CAD build for the part. Positions are in the model's coordinates, mm. A direction names the side the tool comes from. Coordinates: 2 decimals unless noted, no trailing zeros. Order: outer loops, then holes, each group sorted by start corner. A loop starts at its lowest first (then second) coordinate and runs counter-clockwise, first axis right, second up. Notation, with made-up numbers: (40, -16.5) - (68, -16.5) arc R24 ccw to (68, 6.5) - close; hole circle Ø10 at (76.5, 43). An arc over 180 degrees is marked (long way). Return JSON: item names as keys, results as strings.
from build123d import *

# Parameters (mm, degrees)
F1_DEPTH     = 58.3
F3_DEPTH     = 9.017
F4_W         = 5.08
F4_H         = 2.54
F5_DEPTH     = 50.801
F6_T1_DEPTH  = 17.9471724254
F6_T3_DEPTH  = 16.9545
F6_T5_DEPTH  = 52.07
F6_T7_DEPTH  = 22.3848784961
F6_T9_DEPTH  = 12.2248784961
F6_T11_DEPTH = 14.0401215039
F6_T13_DEPTH = 12.5401215039
F6_T16_ANGLE = 90
F6_T18_ANGLE = 90
F6_T20_ANGLE = 90
F6_T22_ANGLE = 90
F7_R         = 5
F8_DEPTH     = 25.4
F9_R         = 2.25
F10_DEPTH    = 49.284


# Not quite as in the source:
# - a fillet or chamfer that OpenCascade refuses, or shapes differently, is made with other operations: its cross-section is extruded or revolved along the edge and cut away or added


with BuildPart() as f1:
    # F0 (on Top) → F1 (new body)
    with BuildSketch(Plane.XY):
        with BuildLine():
            Line((47.625, 58.42), (3.175, 58.42))
            ThreePointArc((3.175, 58.42), (0.9299359697, 57.4900640303), (0, 55.245))
            Line((0, 55.245), (0, 3.175))
            ThreePointArc((0, 3.175), (0.9299359697, 0.9299359697), (3.175, 0))
            Line((3.175, 0), (47.625, 0))
            ThreePointArc((47.625, 0), (49.8700640303, 0.9299359697), (50.8, 3.175))
            Line((50.8, 3.175), (50.8, 55.245))
            ThreePointArc((50.8, 55.245), (49.8700640303, 57.4900640303), (47.625, 58.42))
        make_face()
    extrude(amount=F1_DEPTH)

    # F2 (on face) → F3 (cut)
    with BuildSketch(Plane.XY.offset(58.3)):
        Polygon((33.1776215039, 45.72), (33.1776215039, 58.42), (7.7776215039, 58.42), (7.7776215039, 12.7), (9.2776215039, 0), (43.3376215039, 0), (43.3376215039, 15.24), (48.4176215039, 15.24), (48.4176215039, 30.48), align=None)
    extrude(amount=-F3_DEPTH, mode=Mode.SUBTRACT)

    # F4 (on face) → F5 (cut, through all)
    with BuildSketch(Plane.YZ.offset(50.8)):
        with Locations((15.24, 45.6)):
            Rectangle(F4_W, F4_H)
        with Locations((45.72, 45.6)):
            Rectangle(F4_W, F4_H)
    extrude(amount=-F5_DEPTH, mode=Mode.SUBTRACT)

    # F6: fillet of radius 3.175 on 6 edges, made by hand

    # F6_s2 → F6_t1 (cut)
    with BuildSketch(Plane.XY.offset(49.283)):
        with BuildLine():
            ThreePointArc((5.7055525338, 0), (8.0786339971, 1.0657087996), (8.8586359029, 3.5474114216))
            Line((8.8586359029, 3.5474114216), (9.2776215039, 0))
            Line((9.2776215039, 0), (5.7055525338, 0))
        make_face()
    extrude(amount=F6_T1_DEPTH, mode=Mode.SUBTRACT)

    # F6_s4 → F6_t3 (cut)
    with BuildSketch(Plane.XY.offset(49.283)):
        with BuildLine():
            ThreePointArc((46.5126215039, 0), (44.2675574737, 0.9299359697), (43.3376215039, 3.175))
            Line((43.3376215039, 3.175), (43.3376215039, 0))
            Line((43.3376215039, 0), (46.5126215039, 0))
        make_face()
        with BuildLine():
            ThreePointArc((4.6026215039, 58.42), (6.8476855342, 57.4900640303), (7.7776215039, 55.245))
            Line((7.7776215039, 55.245), (7.7776215039, 58.42))
            Line((7.7776215039, 58.42), (4.6026215039, 58.42))
        make_face()
        with BuildLine():
            ThreePointArc((36.3526215039, 58.42), (34.1075574737, 57.4900640303), (33.1776215039, 55.245))
            Line((33.1776215039, 55.245), (33.1776215039, 58.42))
            Line((33.1776215039, 58.42), (36.3526215039, 58.42))
        make_face()
    extrude(amount=F6_T3_DEPTH, mode=Mode.SUBTRACT)

    # F6_s6 → F6_t5 (cut)
    with BuildSketch(Plane.XZ.offset(-55.245)):
        with BuildLine():
            ThreePointArc((0, 55.125), (0.9299359697, 57.3700640303), (3.175, 58.3))
            Line((3.175, 58.3), (0, 58.3))
            Line((0, 58.3), (0, 55.125))
        make_face()
        with BuildLine():
            ThreePointArc((50.8, 55.125), (49.8700640303, 57.3700640303), (47.625, 58.3))
            Line((47.625, 58.3), (50.8, 58.3))
            Line((50.8, 58.3), (50.8, 55.125))
        make_face()
    extrude(amount=F6_T5_DEPTH, mode=Mode.SUBTRACT)

    # F6_s8 → F6_t7 (cut)
    with BuildSketch(Plane.YZ.offset(25.2401215039)):
        with BuildLine():
            ThreePointArc((55.245, 58.3), (57.4900640303, 57.3700640303), (58.42, 55.125))
            Line((58.42, 55.125), (58.42, 58.3))
            Line((58.42, 58.3), (55.245, 58.3))
        make_face()
    extrude(amount=F6_T7_DEPTH, mode=Mode.SUBTRACT)

    # F6_s10 → F6_t9 (cut)
    with BuildSketch(Plane.YZ.offset(35.4001215039)):
        with BuildLine():
            ThreePointArc((3.175, 58.3), (0.9299359697, 57.3700640303), (0, 55.125))
            Line((0, 55.125), (0, 58.3))
            Line((0, 58.3), (3.175, 58.3))
        make_face()
    extrude(amount=F6_T9_DEPTH, mode=Mode.SUBTRACT)

    # F6_s12 → F6_t11 (cut)
    with BuildSketch(Plane.YZ.offset(3.175)):
        with BuildLine():
            ThreePointArc((0, 55.125), (0.9299359697, 57.3700640303), (3.175, 58.3))
            Line((3.175, 58.3), (0, 58.3))
            Line((0, 58.3), (0, 55.125))
        make_face()
    extrude(amount=F6_T11_DEPTH, mode=Mode.SUBTRACT)

    # F6_s14 → F6_t13 (cut)
    with BuildSketch(Plane.YZ.offset(3.175)):
        with BuildLine():
            ThreePointArc((58.42, 55.125), (57.4900640303, 57.3700640303), (55.245, 58.3))
            Line((55.245, 58.3), (58.42, 58.3))
            Line((58.42, 58.3), (58.42, 55.125))
        make_face()
    extrude(amount=F6_T13_DEPTH, mode=Mode.SUBTRACT)

    # F6_s15 → F6_t16 (revolve, cut)
    with BuildSketch(Plane.YZ.offset(47.625)):
        with BuildLine():
            ThreePointArc((0, 55.125), (0.9299359697, 57.3700640303), (3.175, 58.3))
            Line((3.175, 58.3), (0, 58.3))
            Line((0, 58.3), (0, 55.125))
        make_face()
    revolve(axis=Axis((47.625, 3.175, 58.3), (0, 0, 1)), revolution_arc=F6_T16_ANGLE, mode=Mode.SUBTRACT)

    # F6_s17 → F6_t18 (revolve, cut)
    with BuildSketch(Plane.XZ.offset(-55.245)):
        with BuildLine():
            ThreePointArc((47.625, 58.3), (49.8700640303, 57.3700640303), (50.8, 55.125))
            Line((50.8, 55.125), (50.8, 58.3))
            Line((50.8, 58.3), (47.625, 58.3))
        make_face()
    revolve(axis=Axis((47.625, 55.245, 58.3), (0, 0, 1)), revolution_arc=F6_T18_ANGLE, mode=Mode.SUBTRACT)

    # F6_s19 → F6_t20 (revolve, cut)
    with BuildSketch(Plane.YZ.offset(3.175)):
        with BuildLine():
            ThreePointArc((58.42, 55.125), (57.4900640303, 57.3700640303), (55.245, 58.3))
            Line((55.245, 58.3), (58.42, 58.3))
            Line((58.42, 58.3), (58.42, 55.125))
        make_face()
    revolve(axis=Axis((3.175, 55.245, 58.3), (0, 0, 1)), revolution_arc=F6_T20_ANGLE, mode=Mode.SUBTRACT)

    # F6_s21 → F6_t22 (revolve, cut)
    with BuildSketch(Plane.XZ.offset(-3.175)):
        with BuildLine():
            ThreePointArc((0, 55.125), (0.9299359697, 57.3700640303), (3.175, 58.3))
            Line((3.175, 58.3), (0, 58.3))
            Line((0, 58.3), (0, 55.125))
        make_face()
    revolve(axis=Axis((3.175, 3.175, 58.3), (0, 0, 1)), revolution_arc=F6_T22_ANGLE, mode=Mode.SUBTRACT)

    # F7 (on face) → F8 (cut)
    with BuildSketch(Plane.XY.offset(49.283)):
        with Locations((20.4776215039, 45.72)):
            Circle(F7_R)
        with Locations((30.6376215039, 12.7)):
            Circle(F7_R)
    extrude(amount=-F8_DEPTH, mode=Mode.SUBTRACT)

    # F9 (on face) → F10 (cut, through all)
    with BuildSketch(Plane.XY.offset(49.283)):
        with Locations((20.4776215039, 45.72)):
            Circle(F9_R)
        with Locations((30.6376215039, 12.7)):
            Circle(F9_R)
    extrude(amount=-F10_DEPTH, mode=Mode.SUBTRACT)


solid = f1.part
Item 1: Band-saw the part on A-A, the plane x = 29.5. List the corners of the cut face in (y, z), then the cut area to 3 significant figures.
Findings below:
{"outline": "(0, 0) - (10.76, 0) - (10.76, 23.88) - (7.83, 23.88) - (7.83, 49.28) - (0, 49.28) - close; (14.64, 0) - (58.42, 0) - (58.42, 49.28) - (17.57, 49.28) - (17.57, 46.87) - (17.78, 46.87) - (17.78, 44.33) - (17.57, 44.33) - (17.57, 23.88) - (14.64, 23.88) - close; hole (43.18, 44.33) - (48.26, 44.33) - (48.26, 46.87) - (43.18, 46.87) - close", "area": "2,530 mm²"}
Item 2: Which spindle directions (+Z, -Z, +X, -X, +Y, -Y) get a long thin tool onto all of the face, cutting with end or side? Do faces 1 (the flat face through (40.9, 38, 53.9)), 2 (the flat face through (8, 46, 44.33)), 3 (the cylindrical face through (34.13, 57.51, 53.73)). Say none if no direction does.
Findings below:
{"face 1": "+Z", "face 2": "+X, -X", "face 3": "+Z, +Y"}
Item 3: Band-saw the part on B-B, the plane y = 29.5. List the corners of the cut face in (x, z) (3 decimals).
Findings below:
{"outline": "(0, 0) - (50.8, 0) - (50.8, 55.125) arc R3.175 ccw to (48.418, 58.199) - (48.418, 49.283) - (7.778, 49.283) - (7.778, 58.3) - (3.175, 58.3) arc R3.175 ccw to (0, 55.125) - close"}
Item 4: Wall check: L1, parallel to Z at x = 41.5, y = 17.5; L2, parallel to X at y = 45.72, z = 42.75; L3, parallel to Z at x = 16, y = 52. Give the ranges that are in metal, low to high. Write a range as [from, to].
Findings below:
{"L1": "z = [0, 44.33], [46.87, 49.28]", "L2": "x = [0, 15.48], [25.48, 50.8]", "L3": "z = [0, 49.28]"}
Item 5: Drop flat-ended pins along their axis: P1, Ø3.5, axis at x = 20.48, y = 45.72, coming from the +Z side; P2, Ø11.5, axis at x = 30.64, y = 12.7, coming from the +Z side. Give the stop position or say it passes through.
Findings below:
{"P1": "passes through", "P2": "stops at z = 49.28"}
Item 6: Band-saw the part on C-C, the plane x = 17. List the corners of the cut face in (y, z), then the cut area to 3 significant figures.
Findings below:
{"outline": "(0, 0) - (58.42, 0) - (58.42, 49.28) - (49.31, 49.28) - (49.31, 23.88) - (42.13, 23.88) - (42.13, 49.28) - (0, 49.28) - close; hole (12.7, 44.33) - (17.78, 44.33) - (17.78, 46.87) - (12.7, 46.87) - close", "area": "2,680 mm²"}
Item 7: Mould opens along Y. For faces 4 (the cylindrical face through (6.823, 57.515, 53.728)), 5 (the flat face through (8, 48.26, 46)), 6 (the flat face through (45, 9, 58.3)) say: released by +Y, released by -Y, zero draft, split by the parting line, or undercut.
Findings below:
{"face 4": "released by +Y", "face 5": "undercut", "face 6": "zero draft"}
